Check sheet for the modelled part. Datum: model origin and axes. Units: mm. Give positions to 0.01 mm unless a question says otherwise; leave off trailing zeros. Loops run counter-clockwise (first coordinate to the right, second up) from the corner with the lowest first, then second, coordinate; pieces in that order, holes last. Notation, with made-up numbers: (10, -31.5) -> (50, -31.5) arc R16 ccw to (50, -17.5) -> close; hole circle Ø1 at (72, 25.5). An arc over 180 degrees is marked (long way). Write each question's results on one line, items separated by ' | '. Start each with the question number.
1. Cross-section at B-B on y = 306. Record the boundary of the cut face in (x, z), and give its area (3 significant figures).
2. Material ranges on L1, parallel to Y at x = 0, z = -4.85; L2, parallel to Z at x = -0.5, y = 73, recorded low to high. Write a range as from..to.
3. Cross-section at A-A on x = 0. Record the boundary of the cut face in (y, z), and give its area (3 significant figures).
4. Cross-section at C-C on z = 1.5. Record the boundary of the cut face in (x, y), and give its area (3 significant figures).
from build123d import *

# Parameters (mm, degrees)
CROQUIS1_W              = 10
CROQUIS1_H              = 10
SALIENTE_EXTRUIR1_DEPTH = 500
CROQUIS2_W              = 9.366
CROQUIS2_H              = 9.366
CORTAR_EXTRUIR1_DEPTH   = 500
CROQUIS3_R              = 3
CORTAR_EXTRUIR2_DEPTH   = 500
CROQUIS4_R              = 3
CORTAR_EXTRUIR3_DEPTH   = 500


with BuildPart() as part:
    # Croquis1 → Saliente-Extruir1 (new body)
    with BuildSketch(Plane(origin=(0, 0, 0), x_dir=(1, 0, 0), z_dir=(0, 1, 0))):
        Rectangle(CROQUIS1_W, CROQUIS1_H)
    extrude(amount=SALIENTE_EXTRUIR1_DEPTH)

    # Croquis2 → Cortar-Extruir1 (cut)
    with BuildSketch(Plane(origin=(0, 500, 0), x_dir=(1, 0, 0), z_dir=(0, 1, 0))):
        Rectangle(CROQUIS2_W, CROQUIS2_H)
    extrude(amount=-CORTAR_EXTRUIR1_DEPTH, mode=Mode.SUBTRACT)

    # Croquis3 → Cortar-Extruir2 (cut)
    with BuildSketch(Plane.XY.offset(5)):
        with Locations((0, 5)):
            Circle(CROQUIS3_R)
    extrude(amount=-CORTAR_EXTRUIR2_DEPTH, mode=Mode.SUBTRACT)

    # Croquis4 → Cortar-Extruir3 (cut)
    with BuildSketch(Plane.XY.offset(5)):
        with Locations((0, 495)):
            Circle(CROQUIS4_R)
    extrude(amount=-CORTAR_EXTRUIR3_DEPTH, mode=Mode.SUBTRACT)


solid = part.part
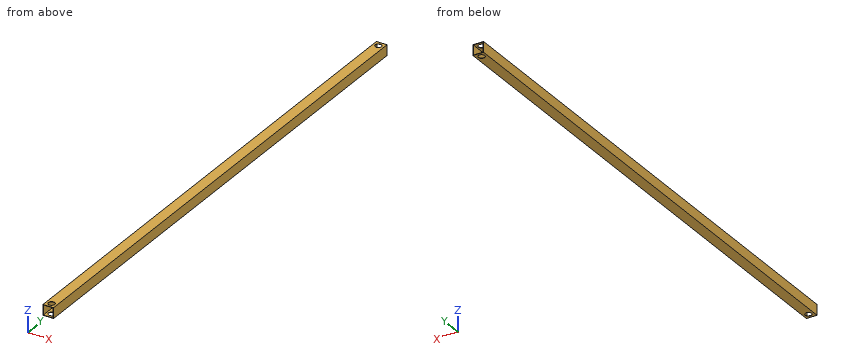
Geometry says:
1) outline: (-5, -5) -> (5, -5) -> (5, 5) -> (-5, 5) -> close; hole (-4.68, -4.68) -> (4.68, -4.68) -> (4.68, 4.68) -> (-4.68, 4.68) -> close | area: 12.3 mm^2
2) L1: 0..2, 8..492, 498..500 | L2: -5..-4.68, 4.68..5
3) outline: (0, -5) -> (2, -5) -> (2, -4.68) -> (0, -4.68) -> close; (0, 4.68) -> (2, 4.68) -> (2, 5) -> (0, 5) -> close; (8, -5) -> (492, -5) -> (492, -4.68) -> (8, -4.68) -> close; (8, 4.68) -> (492, 4.68) -> (492, 5) -> (8, 5) -> close; (498, -5) -> (500, -5) -> (500, -4.68) -> (498, -4.68) -> close; (498, 4.68) -> (500, 4.68) -> (500, 5) -> (498, 5) -> close | area: 309 mm^2
4) outline: (-5, 0) -> (-4.68, 0) -> (-4.68, 500) -> (-5, 500) -> close; (4.68, 0) -> (5, 0) -> (5, 500) -> (4.68, 500) -> close | area: 317 mm^2
